Read the model definition and answer for the solid it produces. Units are mm, in the model's axes. A direction names the side the tool comes from. Coordinates: 2 decimals unless noted, no trailing zeros. Order: outer loops, then holes, each group sorted by start corner. A loop starts at its lowest first (then second) coordinate and runs counter-clockwise, first axis right, second up. Notation, with made-up numbers: (-36.5, 32) -> (5.5, 32) arc R12 cw to (5.5, 48) -> close; hole circle Ø4 at (43, 64). An arc over 180 degrees is marked (long way). Answer in a Markdown table with one row per item.
from build123d import *

# Parameters (mm, degrees)
ESBO_O1_W                = 43
ESBO_O1_H                = 43
RESSALTO_EXTRUS_O1_DEPTH = 3
ESBO_O2_W                = 43
ESBO_O2_H                = 3
RESSALTO_EXTRUS_O2_DEPTH = 46
ESBO_O3_R                = 1.75
CORTE_EXTRUS_O1_DEPTH    = 56.140729048
ESBO_O4_R                = 1.75
CORTE_EXTRUS_O2_DEPTH    = 69.645830172
RESSALTO_EXTRUS_O3_DEPTH = 3
RESSALTO_EXTRUS_O4_DEPTH = 3
ESBO_O7_R                = 12.25
CORTE_EXTRUS_O3_DEPTH    = 3
FILETE1_R                = 3.5
FILETE2_R                = 7
FILETE3_R                = 3.5
FILETE4_R                = 5
ESBO_O8_W                = 16
ESBO_O8_H                = 8
CORTE_EXTRUS_O4_DEPTH    = 57.378187353
FILETE5_R                = 1


with BuildPart() as part:
    # Esboço1 → Ressalto-extrusão1 (new body)
    with BuildSketch(Plane(origin=(0, 0, 0), x_dir=(1, 0, 0), z_dir=(0, 1, 0))):
        Rectangle(ESBO_O1_W, ESBO_O1_H)
    extrude(amount=RESSALTO_EXTRUS_O1_DEPTH)

    # Esboço2 → Ressalto-extrusão2 (add)
    with BuildSketch(Plane(origin=(0, 3, 0), x_dir=(1, 0, 0), z_dir=(0, 1, 0))):
        with Locations((0, -20)):
            Rectangle(ESBO_O2_W, ESBO_O2_H)
    extrude(amount=RESSALTO_EXTRUS_O2_DEPTH)

    # Esboço3 → Corte-extrusão1 (cut, through all)
    with BuildSketch(Plane(origin=(0, 3, 0), x_dir=(1, 0, 0), z_dir=(0, 1, 0))):
        with Locations(Location((14.945, 12.03, 0), (0, 0, 270))):
            Circle(ESBO_O3_R)
        with Locations(Location((14.945, -12.03, 0), (0, 0, 90))):
            Circle(ESBO_O3_R)
        with Locations(Location((-14.945, -12.03, 0), (0, 0, 270))):
            Circle(ESBO_O3_R)
        with Locations(Location((-14.945, 12.03, 0), (0, 0, 90))):
            Circle(ESBO_O3_R)
    extrude(amount=-CORTE_EXTRUS_O1_DEPTH, mode=Mode.SUBTRACT)

    # Esboço4 → Corte-extrusão2 (cut, through all)
    with BuildSketch(Plane.XY.offset(21.5)):
        with Locations((-15.5, 43)):
            Circle(ESBO_O4_R)
        with Locations((15.5, 43)):
            Circle(ESBO_O4_R)
        with Locations((-15.5, 12)):
            Circle(ESBO_O4_R)
        with Locations((15.5, 12)):
            Circle(ESBO_O4_R)
    extrude(amount=-CORTE_EXTRUS_O2_DEPTH, mode=Mode.SUBTRACT)

    # Esboço5 → Ressalto-extrusão3 (add)
    with BuildSketch(Plane.ZY.offset(21.5)):
        Polygon((-21.5, 0), (-21.5, 3), (18.5, 49), (21.5, 49), (21.5, 0), align=None)
    extrude(amount=RESSALTO_EXTRUS_O3_DEPTH)

    # Esboço6 → Ressalto-extrusão4 (add)
    with BuildSketch(Plane(origin=(21.5, 0, 0), x_dir=(0, 0, -1), z_dir=(1, 0, 0))):
        Polygon((21.5, 0), (-21.5, 0), (-21.5, 49), (-18.5, 49), (21.5, 3), align=None)
    extrude(amount=RESSALTO_EXTRUS_O4_DEPTH)

    # Esboço7 → Corte-extrusão3 (cut)
    with BuildSketch(Plane.XY.offset(21.5)):
        with Locations((0, 27.5)):
            Circle(ESBO_O7_R)
    extrude(amount=-CORTE_EXTRUS_O3_DEPTH, mode=Mode.SUBTRACT)

    # Filete1
    # the kernel refuses this fillet: 3.5 mm, written as the material it takes off along each edge
    with BuildSketch(Plane(origin=(-24.5, 49, 9.75), x_dir=(1, 0, 0), z_dir=(0, 0, 1)), Plane(origin=(24.5, 49, 30.25), x_dir=(-1, 0, 0), z_dir=(0, 0, -1))) as filete1_piece_1:
        with BuildLine():
            CenterArc((FILETE1_R, -FILETE1_R), FILETE1_R, 90, 90)
            Line((0, -FILETE1_R), (0, 0))
            Line((0, 0), (FILETE1_R, 0))
        make_face()
    extrude(amount=20.5, mode=Mode.SUBTRACT)

    # Filete2
    filete2_edges = [part.edges().sort_by_distance(p)[0] for p in [
        (0, 0, 21.5),
    ]]
    fillet(filete2_edges, radius=FILETE2_R)

    # Filete3
    # the kernel refuses this fillet: 3.5 mm, written as the material it takes off along each edge
    with BuildSketch(Plane(origin=(-24.5, -8.75, -21.5), x_dir=(0, 0, 1), z_dir=(0, 1, 0)), Plane(origin=(24.5, 11.75, -21.5), x_dir=(0, 0, 1), z_dir=(0, -1, 0))) as filete3_piece_1:
        with BuildLine():
            CenterArc((FILETE3_R, FILETE3_R), FILETE3_R, 180, 90)
            Line((0, FILETE3_R), (0, 0))
            Line((0, 0), (FILETE3_R, 0))
        make_face()
    extrude(amount=20.5, mode=Mode.SUBTRACT)

    # Filete4
    filete4_edges = [part.edges().sort_by_distance(p)[0] for p in [
        (0, 3, 18.5),
    ]]
    fillet(filete4_edges, radius=FILETE4_R)

    # Esboço8 → Corte-extrusão4 (cut, through all)
    with BuildSketch(Plane(origin=(0, 3, 0), x_dir=(1, 0, 0), z_dir=(0, 1, 0))):
        with Locations((0, 17.5)):
            Rectangle(ESBO_O8_W, ESBO_O8_H)
    extrude(amount=-CORTE_EXTRUS_O4_DEPTH, mode=Mode.SUBTRACT)

    # Filete5
    filete5_edges = [part.edges().sort_by_distance(p)[0] for p in [
        (-8, 1.5, -21.5),
        (8, 1.5, -21.5),
        (8, 1.5, -13.5),
        (-8, 1.5, -13.5),
    ]]
    fillet(filete5_edges, radius=FILETE5_R)


solid = part.part
Q1. The part is cut by section A-A (z = -16). Write down the section's boundary in (x, y) (3 decimals).
Outcome:
| item | result |
|---|---|
| outline | (-24.5, 0) -> (-8, 0) -> (-8, 3) -> (-21.5, 3) -> (-21.5, 9.325) -> (-24.5, 9.325) -> close; (8, 0) -> (24.5, 0) -> (24.5, 9.325) -> (21.5, 9.325) -> (21.5, 3) -> (8, 3) -> close |
Q2. The part is cut by section C-C (y = 42). Write down the section's boundary in (x, z), then the cut area to 3 significant figures.
Outcome:
| item | result |
|---|---|
| outline | (-24.5, 12.41) -> (-21.5, 12.41) -> (-21.5, 18.5) -> (-16.94, 18.5) -> (-16.94, 21.5) -> (-24.5, 21.5) -> close; (-14.06, 18.5) -> (14.06, 18.5) -> (14.06, 21.5) -> (-14.06, 21.5) -> close; (16.94, 18.5) -> (21.5, 18.5) -> (21.5, 12.41) -> (24.5, 12.41) -> (24.5, 21.5) -> (16.94, 21.5) -> close |
| area | 166 mm² |
Q3. The part is cut by section B-B (x = 0). Write down the section's boundary in (y, z).
Outcome:
| item | result |
|---|---|
| outline | (0, -13.5) -> (3, -13.5) -> (3, 13.5) arc R5 cw to (8, 18.5) -> (15.25, 18.5) -> (15.25, 21.5) -> (7, 21.5) arc R7 ccw to (0, 14.5) -> close; (39.75, 18.5) -> (49, 18.5) -> (49, 21.5) -> (39.75, 21.5) -> close |
Q4. Given pin 1 (12.5 mm diameter, centred on x = -3, y = 35, fed in from -Z); pin 2 (4 mm diameter, centred on x = -6.5, z = 0.5, fed in from +Y), each flat-ended and moving along its own axis, determine where each tip first touches the part or whether it passes through.
Outcome:
| item | result |
|---|---|
| pin 1 | z = 18.5 |
| pin 2 | y = 3 |
Q5. Consider line 1 (X direction, y = 1, z = 12); line 2 (X direction, y = 9, z = -2.5); line 3 (Z direction, x = 13, y = 25). Determine where each line is inside the solid, lowest interval first.
Outcome:
| item | result |
|---|---|
| line 1 | -24.5 to -16.69, -13.2 to 13.2, 16.69 to 24.5 |
| line 2 | -24.5 to -21.5, 21.5 to 24.5 |
| line 3 | 18.5 to 21.5 |
Q6. The part is cut by section D-D (z = 12.03). Write down the section's boundary in (x, y) (1 decimal).
Outcome:
| item | result |
|---|---|
| outline | (-24.5, 0) -> (-16.7, 0) -> (-16.7, 3) -> (-21.5, 3) -> (-21.5, 41.6) -> (-24.5, 41.6) -> close; (-13.2, 0) -> (13.2, 0) -> (13.2, 3) -> (-13.2, 3) -> close; (16.7, 0) -> (24.5, 0) -> (24.5, 41.6) -> (21.5, 41.6) -> (21.5, 3) -> (16.7, 3) -> close |
Q7. For faces 1 (the face through (0, 49, 20)), 2 (the face through (-18.66, 4.43, 17)), 3 (the face through (8, 2, -17)), determine the directions among +Z, -Z, +X, -X, +Y, -Y from which every point of the face is accessible in a straight line to the end or side of a thin tool.
Outcome:
| item | result |
|---|---|
| face 1 | +Z, -Z, +X, -X, +Y |
| face 2 | -Z, +Y |
| face 3 | -Z, +Y, -Y |
Q8. For a pull along Y with two mould halves and no side action, classify faces 4 (the face through (17.169, 12.526, 20.021)), 5 (the face through (0, 2, -13.5)), 6 (the face through (15.12, 41.29, 20.02)), 7 (the face through (0, 3, -4)) as pulls with the +Y half, pulls with the -Y half, needs draft (parallel to the pull), parting line crosses it, or undercut.
Outcome:
| item | result |
|---|---|
| face 4 | undercut |
| face 5 | needs draft |
| face 6 | undercut |
| face 7 | pulls with the +Y half |
